Can you work these out from the drawing? Everything is in mm from the part's minimum corner. A direction names the side the tool comes from. Coordinates: 2 decimals unless noted, no trailing zeros. Order: outer loops, then holes, each group sorted by start corner. A loop starts at its lowest first (then second) coordinate and runs counter-clockwise, first axis right, second up. Notation, with made-up numbers: (77, 2.5) - (100, 2.5) arc R19 cw to (100, 29.5) - close; hole circle Ø8 at (18.5, -34). An arc over 180 degrees is marked (long way). Use a Markdown table: item, result. Add a question column.
(1) We'd pull the mould along Y, two halves only. Please class the marked faces 1, 2 and 3: pulls with the +Y half, pulls with the -Y half, needs draft (parallel to the pull), parting line crosses it, or undercut.
(2) I want a section at B-B (y = 25.4). List the corners of the cut face in (x, z) for me.
(3) For pin 1 Ø2.5 at (x, y) = (7.239, 25.4) entering from +Z; pin 2 Ø3.5 at (x, z) = (16.5, 3.5) entering from -Y; pin 3 Ø1.9 at (y, z) = (45, 4) entering from +X, each with a flat end and sliding along its axis, tell me the tip position at first contact or that it passes through.
(4) If I drill on L1, parallel to Y at x = 7.25, z = 0.5; L2, parallel to Y at x = 17.75, z = 6; L3, parallel to X at y = 2, z = 6, over which ranges is the centre line in solid material (lowest first)? Write a range as [from, to].
(5) I want a section at C-C (z = 5.25). State how many separate pieces and enclosed holes the cut face has, and give its area (3 significant figures).
(6) I want a section at A-A (x = 15). List the corners of the cut face in (y, z) for me, and give its area (3 significant figures).
(7) On a 3-axis mill with a long thin cutter (end or side, diameter ignored), from which of +Z, -Z, +X, -X, +Y, -Y can I reach the whole of each face in a straight line? I mean the marked faces 4, 5, 6 and 7. Say none if no direction works.
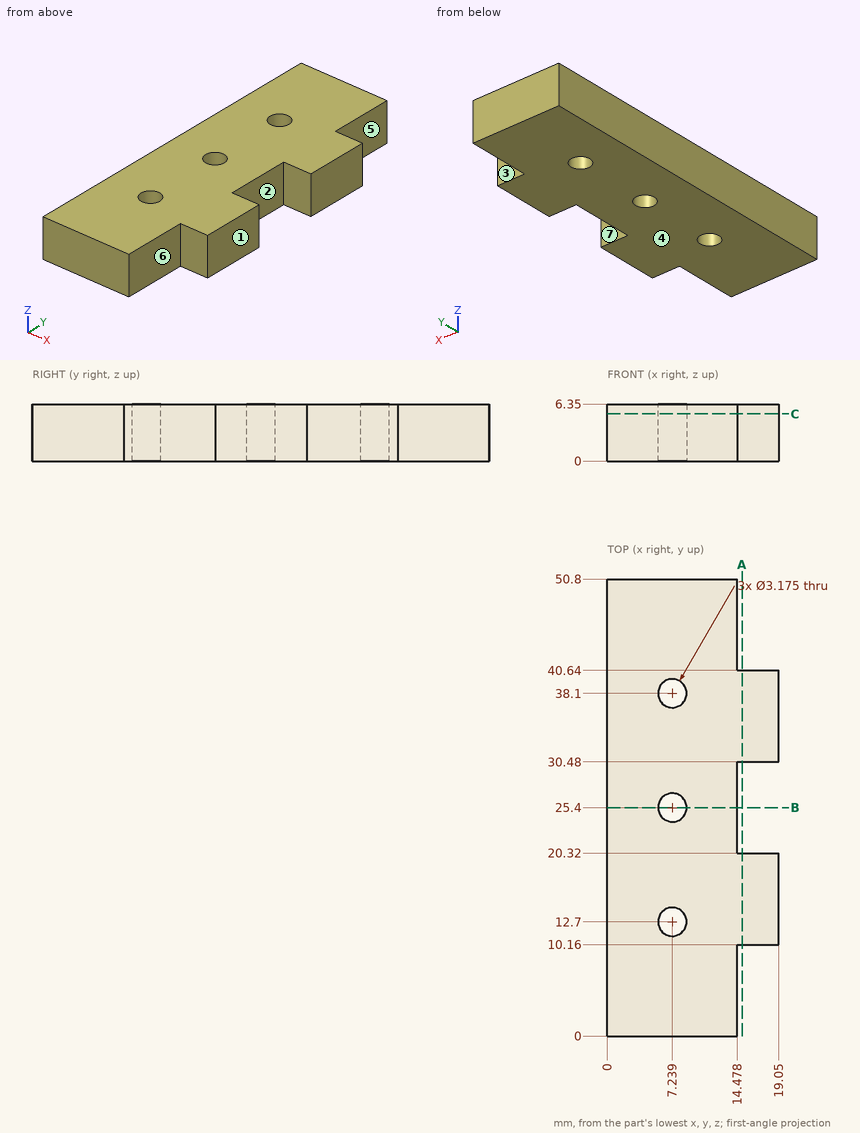
Answers follow:
| question | item | result |
|---|---|---|
| 1 | face 1 | needs draft |
| 1 | face 2 | undercut |
| 1 | face 3 | pulls with the +Y half |
| 2 | outline | (0, 0) - (5.65, 0) - (5.65, 6.35) - (0, 6.35) - close; (8.83, 0) - (14.48, 0) - (14.48, 6.35) - (8.83, 6.35) - close |
| 3 | pin 1 | passes through |
| 3 | pin 2 | stops at y = 10.16 |
| 3 | pin 3 | stops at x = 14.48 |
| 4 | L1 | y = [0, 11.11], [14.29, 23.81], [26.99, 36.51], [39.69, 50.8] |
| 4 | L2 | y = [10.16, 20.32], [30.48, 40.64] |
| 4 | L3 | x = [0, 14.48] |
| 5 | separate pieces | 1 |
| 5 | enclosed holes | 3 |
| 5 | area | 805 mm² |
| 6 | outline | (10.16, 0) - (20.32, 0) - (20.32, 6.35) - (10.16, 6.35) - close; (30.48, 0) - (40.64, 0) - (40.64, 6.35) - (30.48, 6.35) - close |
| 6 | area | 129 mm² |
| 7 | face 4 | -Z, +X, -X, +Y, -Y |
| 7 | face 5 | +Z, -Z, +X, +Y |
| 7 | face 6 | +Z, -Z, +X, -Y |
| 7 | face 7 | +Z, -Z, +X |
